Geometry check sheet. Reference: the model listing, model coordinates, mm. A direction names the side the tool comes from. Give positions to 0.01 mm unless a question says otherwise; leave off trailing zeros. Order: outer loops, then holes, each group sorted by start corner. A loop starts at its lowest first (then second) coordinate and runs counter-clockwise, first axis right, second up. Notation, with made-up numbers: M -21,-0.5 L 12,-0.5 A15 cw 12,3.5 Z; hole C -24,87 d3. An arc over 180 degrees is marked long. Put each result on its own line as item: value. Start each with the question number.
Q1. Mould release check, pull along Y, two halves, no side actions. Record for faces 4 (the cylindrical face through (31.5, 9.9, 93.6)), 5 (the cylindrical face through (-0.794, 6.044, 127.631)), 6 (the flat face through (-27.1, -17.3, 67.831)): +Y half, -Y half, draft (parallel to the pull), parting line (faces both ways), or undercut.
Q2. Material ranges on L1, parallel to X at y = 0, z = 124.5; L2, parallel to Y at x = 0, z = 85; L3, parallel to Z at x = -11, y = 27, recorded low to high.
Q3. Section check A-A on x = 0. Record the cut outline in (y, z), then the cut area to 3 significant figures.
Q4. Access from +Z, -Z, +X, -X, +Y, -Y to the whole of each face (thin tool, end or side, straight path). Record for faces 1 (the cylindrical face through (29.44, -12.2, 94.46)), 2 (the cylindrical face through (-4.82, -23.14, 122.27)), 3 (the cylindrical face through (-1.38, -6.2, 127.9)).
Q5. Section check C-C on y = -4. State how many separate pieces and enclosed holes the cut face has, then the cut area to 3 significant figures.
Q6. Go/stop test with flat-tipped pins: pin 1 (2 mm diameter, centred on x = -19, y = 8.5, fed in from +Z); pin 2 (14.5 mm diameter, centred on x = -0.29, y = 20.18, fed in from -Z); pin 3 (12 mm diameter, centred on x = -18.5, z = 124.5, fed in from +Y); pin 4 (11 mm diameter, centred on x = 0, y = 0, fed in from +Z). Record where each tip stops, or that it passes through.
Q7. Section check B-B on z = 79. Record the cut outline in (x, y).
```python
from build123d import *

# Parameters (mm, degrees)
F0_R           = 27.051
F2_R           = 33.02
F4_DEPTH       = 112.522
F8_DEPTH       = 25.4
F6_R           = 31.8662185307
F10_R          = 27.1012036097
F12_DEPTH      = 111.67649
F13_R          = 6.35
F13_R_2        = 6.096
F14_DEPTH      = 25.4
F15_DEPTH      = 25.4
F16_W          = 95.3798592091
F16_H          = 79.9988703802
F17_DEPTH      = 50.8
F17_DEPTH_BACK = 50.8
F18_R          = 4.5084907347
F18_R_2        = 5.1462074836
F18_R_3        = 5.3392585876
F18_R_4        = 2.9616888365
F19_DEPTH      = 25.4
F20_R          = 2.54
F21_W          = 29.3621988967
F21_H          = 16.516238451
F22_DEPTH      = 25.4
F22_DEPTH_BACK = 25.4


with BuildPart() as f3:
    # F0 (on Top) → F3 section 0
    with BuildSketch(Plane.XY):
        Circle(F0_R)
    # F2 (on offset) → F3 section 1
    with BuildSketch(Plane.XY.offset(10.16)):
        Circle(F2_R)
    loft()

    # F4 (add): a face of the model
    f4_faces = [f3.faces().sort_by_distance(p)[0] for p in [
        (0, 0, 10.16),
    ]]
    extrude(f4_faces, amount=F4_DEPTH)

    # F7 (on face) → F8 (cut)
    with BuildSketch(Plane(origin=(0, 0, 0), x_dir=(1, 0, 0), z_dir=(0, 0, -1))):
        with BuildLine():
            Line((-9.0020672118, 14.5257171748), (8.9738084456, 14.5257171748))
            ThreePointArc((8.9738084456, 14.5257171748), (-0.0141293831, 22.7222466067), (-9.0020672118, 14.5257171748))
        make_face()
    extrude(amount=-F8_DEPTH, mode=Mode.SUBTRACT)

    # F6 (on offset) → F11 section 0
    with BuildSketch(Plane.XY.offset(10.16)):
        Circle(F6_R)
    # F10 (on offset) → F11 section 1
    with BuildSketch(Plane(origin=(0, 0, 1.016), x_dir=(1, 0, 0), z_dir=(0, 0, -1))):
        Circle(F10_R)
    loft(mode=Mode.SUBTRACT)

    # F6 (on offset) → F12 (cut)
    with BuildSketch(Plane.XY.offset(10.16)):
        Circle(F6_R)
    extrude(amount=F12_DEPTH, mode=Mode.SUBTRACT)

    # F13 (on face) → F14 (join)
    with BuildSketch(Plane.XY.offset(122.682)):
        Circle(F13_R)
        Circle(F13_R_2, mode=Mode.SUBTRACT)
    extrude(amount=F14_DEPTH)

    # F15 (cut): a face of the model
    f15_faces = [f3.faces().sort_by_distance(p)[0] for p in [
        (0, 0, 122.682),
    ]]
    extrude(f15_faces, amount=-F15_DEPTH, mode=Mode.SUBTRACT)

    # F16 (on Right) → F17 (cut, two sides)
    with BuildSketch(Plane.YZ) as f17_sk:
        with Locations((3.9506442845, 27.8317159973)):
            Rectangle(F16_W, F16_H)
    extrude(amount=-F17_DEPTH, mode=Mode.SUBTRACT)
    extrude(f17_sk.sketch, amount=F17_DEPTH_BACK, mode=Mode.SUBTRACT)

    # F18 (on face) → F19 (cut)
    with BuildSketch(Plane.XY.offset(122.682)):
        with Locations((-0.2904168505, 20.1840121299)):
            Circle(F18_R)
        with Locations((21.2004743516, -0.7260435959)):
            Circle(F18_R_2)
        with Locations((-0.5808342248, -19.8935940862)):
            Circle(F18_R_3)
        with Locations((-21.7813067138, 2.4685480166)):
            Circle(F18_R_4)
    extrude(amount=-F19_DEPTH, mode=Mode.SUBTRACT)

    # F20
    f20_edges = [f3.edges().sort_by_distance(p)[0] for p in [
        (-33.02, 0, 122.682),
    ]]
    fillet(f20_edges, radius=F20_R)

    # F21 (on Front) → F22 (cut, two sides)
    with BuildSketch(Plane.XZ) as f22_sk:
        with Locations((0.4587839358, 141.5242999792)):
            Rectangle(F21_W, F21_H)
    extrude(amount=-F22_DEPTH, mode=Mode.SUBTRACT)
    extrude(f22_sk.sketch, amount=F22_DEPTH_BACK, mode=Mode.SUBTRACT)


solid = f3.part
```
Results found:
1. face 4: parting line
1. face 5: undercut
1. face 6: draft
2. L1: x = -6.35 to -6.1, 6.1 to 6.35
2. L2: y = -33.02 to -31.87, 31.87 to 33.02
2. L3: z = 121.84 to 122.68
3. outline: M -33.02,67.83 L -31.87,67.83 L -31.87,121.84 L -25.2,121.84 L -25.2,122.68 L -30.48,122.68 A2.54 ccw -33.02,120.14 Z; M -14.59,121.84 L -6.1,121.84 L -6.1,133.27 L -6.35,133.27 L -6.35,122.68 L -14.59,122.68 Z; M 6.1,121.84 L 15.68,121.84 L 15.68,122.68 L 6.35,122.68 L 6.35,133.27 L 6.1,133.27 Z; M 24.68,121.84 L 31.87,121.84 L 31.87,67.83 L 33.02,67.83 L 33.02,120.14 A2.54 ccw 30.48,122.68 L 24.68,122.68 Z
3. area: 156 mm^2
4. face 1: -Z
4. face 2: +Z, -Z
4. face 3: +Z
5. separate pieces: 3
5. enclosed holes: 0
5. area: 171 mm^2
6. pin 1: stops at z = 122.68
6. pin 2: stops at z = 121.84
6. pin 3: stops at y = 29.92
6. pin 4: passes through
7. outline: C 0,0 d66.04; hole C 0,0 d63.73
